Check sheet for the modelled part. Datum: model origin and axes. Units: mm. A direction names the side the tool comes from. Round coordinates to 2 decimals unless told otherwise and drop trailing zeros. Order: outer loops, then holes, each group sorted by start corner. A loop starts at its lowest first (then second) coordinate and runs counter-clockwise, first axis right, second up. Notation, with made-up numbers: (44, 57) -> (83, 57) arc R10 cw to (83, 76) -> close; hole circle Ø1 at (-12.75, 88). An arc over 180 degrees is marked (long way). Answer in a Markdown table with one row per item. Add a question column.
1. Material ranges on L1, parallel to X at y = 17, z = 1.15; L2, parallel to Y at x = -34, z = 1.35; L3, parallel to X at y = 19.5, z = 1.35, recorded low to high. Write a range as from..to.
2. Sectioned sample at C-C, the plane y = 6. Record the boundary of the cut face in (x, z), then the cut area to 3 significant figures.
3. Sectioned sample at A-A, the plane z = 1.35. Record the boundary of the cut face in (x, y).
4. Sectioned sample at B-B, the plane x = 24. Record the boundary of the cut face in (y, z), then the cut area to 3 significant figures.
5. Depth check by flat-ended pin: P1, Ø0.8, axis at x = -7.5, z = 0.5, coming from the +Y side. Enter the tip coordinate at first touch or a pass-through.
6. Access from +Z, -Z, +X, -X, +Y, -Y to the whole of each face (thin tool, end or side, straight path). Record for faces 1 (the flat face through (-9, 2.611, 1)), 2 (the flat face through (0, -6, 0)).
```python
from build123d import *

# Parameters (mm, degrees)
F1_DEPTH = 2.54


with BuildPart() as f1:
    # F0 (on Top) → F1 (new body)
    with BuildSketch(Plane.XY):
        with BuildLine():
            Line((52.056518, 2.611155), (-72.403482, 2.611155))
            ThreePointArc((-72.403482, 2.611155), (-74.199533, 1.867206), (-74.943482, 0.071155))
            Line((-74.943482, 0.071155), (-74.943482, -13.898845))
            ThreePointArc((-74.943482, -13.898845), (-74.199533, -15.694897), (-72.403482, -16.438845))
            Line((-72.403482, -16.438845), (74.916518, -16.438845))
            ThreePointArc((74.916518, -16.438845), (76.712569, -15.694897), (77.456518, -13.898845))
            Line((77.456518, -13.898845), (77.456518, 2.611155))
            Line((77.456518, 2.611155), (77.456518, 19.121155))
            ThreePointArc((77.456518, 19.121155), (76.712569, 20.917206), (74.916518, 21.661155))
            Line((74.916518, 21.661155), (54.596518, 21.661155))
            ThreePointArc((54.596518, 21.661155), (52.800467, 20.917206), (52.056518, 19.121155))
            Line((52.056518, 19.121155), (52.056518, 2.611155))
        make_face()
    extrude(amount=F1_DEPTH)


solid = f1.part
```
Answer key:
| question | item | result |
|---|---|---|
| 1 | L1 | x = 52.06..77.46 |
| 1 | L2 | y = -16.44..2.61 |
| 1 | L3 | x = 52.08..77.43 |
| 2 | outline | (52.06, 0) -> (77.46, 0) -> (77.46, 2.54) -> (52.06, 2.54) -> close |
| 2 | area | 64.5 mm² |
| 3 | outline | (-74.94, -13.9) arc R2.54 ccw to (-72.4, -16.44) -> (74.92, -16.44) arc R2.54 ccw to (77.46, -13.9) -> (77.46, 19.12) arc R2.54 ccw to (74.92, 21.66) -> (54.6, 21.66) arc R2.54 ccw to (52.06, 19.12) -> (52.06, 2.61) -> (-72.4, 2.61) arc R2.54 ccw to (-74.94, 0.07) -> close |
| 4 | outline | (-16.44, 0) -> (2.61, 0) -> (2.61, 2.54) -> (-16.44, 2.54) -> close |
| 4 | area | 48.4 mm² |
| 5 | P1 | stops at y = 2.61 |
| 6 | face 1 | +Z, -Z, -X, +Y |
| 6 | face 2 | -Z, +X, -X, +Y, -Y |
